Check sheet for the modelled part. Datum: model origin and axes. Units: mm. Give positions to 0.01 mm unless a question says otherwise; leave off trailing zeros. Order: outer loops, then holes, each group sorted by start corner. A loop starts at its lowest first (then second) coordinate and runs counter-clockwise, first axis right, second up.
from build123d import *

# Parameters (mm, degrees)
BOSS_EXTRUDE1_DEPTH = 35.56
CUT_EXTRUDE1_DEPTH  = 2.54


with BuildPart() as part:
    # Sketch1 → Boss-Extrude1 (new body)
    with BuildSketch(Plane(origin=(0, 0, 0), x_dir=(1, 0, 0), z_dir=(0, 1, 0))):
        with BuildLine():
            Line((-67.31, -97.79), (67.31, -97.79))
            ThreePointArc((67.31, -97.79), (88.862614691, -88.862614691), (97.79, -67.31))
            Line((97.79, -67.31), (97.79, 67.31))
            ThreePointArc((97.79, 67.31), (88.862614691, 88.862614691), (67.31, 97.79))
            Line((67.31, 97.79), (-67.31, 97.79))
            ThreePointArc((-67.31, 97.79), (-88.862614691, 88.862614691), (-97.79, 67.31))
            Line((-97.79, 67.31), (-97.79, -67.31))
            ThreePointArc((-97.79, -67.31), (-88.862614691, -88.862614691), (-67.31, -97.79))
        make_face()
    extrude(amount=BOSS_EXTRUDE1_DEPTH)

    # Sketch2 → Cut-Extrude1 (cut)
    with BuildSketch(Plane(origin=(0, 35.56, 0), x_dir=(1, 0, 0), z_dir=(0, 1, 0))):
        with BuildLine():
            add(Edge.make_bspline(
                [(1.069159263, 12.053957352), (7.026900295, 11.625396007), (25.310862844, 29.234177767), (30.491031338, -7.916988095), (15.026759827, -36.109498005), (1.530770275, -21.83529591), (-6.040576613, -30.612635114), (-20.658401128, -26.846483994), (-28.267746675, -2.501714901), (-10.902260805, -7.058320175), (-14.044140154, 10.399607654), (-25.914455938, 3.072974608), (-29.507731033, 20.421135825), (-10.125556887, 21.796230615), (-3.363362348, 12.372804279), (1.069159263, 12.053957352)],
                knots=[0, 0, 0, 0, 0.107274199, 0.250434142, 0.395980258, 0.443398128, 0.47894856, 0.546712741, 0.653285311, 0.68880468, 0.749021257, 0.788585463, 0.841034552, 0.920188675, 1, 1, 1, 1], degree=3))
        make_face()
        with BuildLine():
            add(Edge.make_bspline(
                [(4.288165985, 31.968571753), (4.959875783, 32.927739875), (13.302817449, 26.054551709), (5.976088668, 17.468338472), (-5.163355857, 24.084090932), (7.583617977, 23.014813046), (3.679789011, 31.099839749), (4.288165985, 31.968571753)],
                knots=[0, 0, 0, 0, 0.21621725, 0.454945614, 0.634777537, 0.804169008, 1, 1, 1, 1], degree=3))
        make_face()
    extrude(amount=-CUT_EXTRUDE1_DEPTH, mode=Mode.SUBTRACT)


solid = part.part
1) Section check A-A, the plane y = 9. Record the cut outline in (x, z).
Recorded:
outline: (-97.79, -67.31) arc R30.48 ccw to (-67.31, -97.79) - (67.31, -97.79) arc R30.48 ccw to (97.79, -67.31) - (97.79, 67.31) arc R30.48 ccw to (67.31, 97.79) - (-67.31, 97.79) arc R30.48 ccw to (-97.79, 67.31) - close
2) Section check C-C, the plane x = -84. Record the cut outline in (y, z).
Recorded:
outline: (0, -92.81) - (35.56, -92.81) - (35.56, 92.81) - (0, 92.81) - close
3) Draft check along X on faces 1 (the face through (1, 18, -97.79)), 2 (the face through (89.1, 17.53, -88.62)), 3 (the face through (1, 33.02, 3)), 4 (the face through (-89.1, 17.53, 88.62)). Enter one of: +X half, -X half, draft (parallel to the pull), parting line (faces both ways), or undercut.
Recorded:
face 1: draft
face 2: +X half
face 3: undercut
face 4: -X half
4) Section check B-B, the plane z = -79.5. Record the cut outline in (x, y), then the cut area to 3 significant figures.
Recorded:
outline: (-95.25, 0) - (95.25, 0) - (95.25, 35.56) - (-95.25, 35.56) - close
area: 6,770 mm2
5) Depth check by flat-ended pin: pin 1 Ø10 at (x, y) = (-77.5, 7.5) entering from +Z; pin 2 Ø12.5 at (x, z) = (6, -26) entering from +Y; pin 3 Ø12 at (y, z) = (23, -77.5) entering from +X. Enter the tip coordinate at first touch or a pass-through.
Recorded:
pin 1: stops at z = 97.34
pin 2: stops at y = 35.56
pin 3: stops at x = 97.5
6) Material ranges on L1, parallel to Z at x = -67.5, y = 5; L2, parallel to Z at x = -74.5, y = 10.5, recorded low to high.
Recorded:
L1: z = -97.79 to 97.79
L2: z = -96.93 to 96.93
